For this review, take the finished solid that the model builds, in its own axes (mm). Face numbers are marked on the shaded views. Coordinates: 2 decimals unless noted, no trailing zeros. Loops run counter-clockwise (first coordinate to the right, second up) from the corner with the lowest first, then second, coordinate; pieces in that order, holes last.
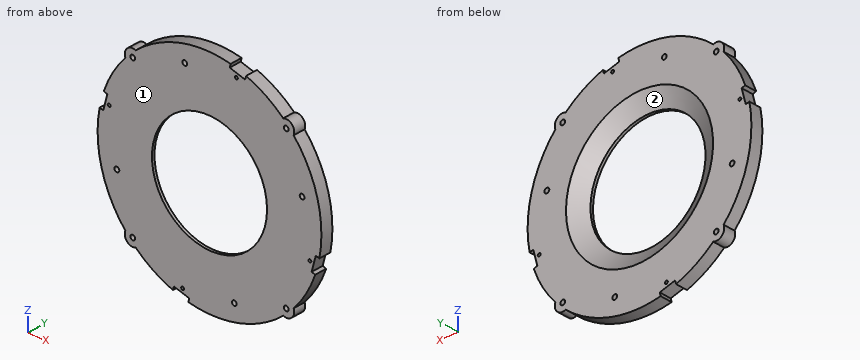
```python
from build123d import *

# Parameters (mm, degrees)
SKETCH1_R           = 1.905
BOSS_EXTRUDE1_DEPTH = 9.525
SKETCH2_R           = 45.72
CUT_EXTRUDE1_DEPTH  = 12.7
SKETCH10_R          = 0.6985
CUT_EXTRUDE5_DEPTH  = 3.175
CIRPATTERN5_COUNT   = 4
CHAMFER1_SIZE       = 12.7
CHAMFER1_SIZE2      = 7.332348419
SKETCH4_R           = 1.905
CUT_EXTRUDE6_DEPTH  = 10.5250001
CIRPATTERN6_COUNT   = 4
SKETCH13_R          = 1.1303
CUT_EXTRUDE7_DEPTH  = 10.5250001
CIRPATTERN7_COUNT   = 4
SKETCH14_W          = 11.95230377
SKETCH14_H          = 12.7
CUT_EXTRUDE8_DEPTH  = 3.175
CIRPATTERN8_COUNT   = 4


with BuildPart() as part:
    # Sketch1 → Boss-Extrude1 (new body)
    with BuildSketch(Plane(origin=(0, 0, 0), x_dir=(1, 0, 0), z_dir=(0, 1, 0))):
        with BuildLine():
            ThreePointArc((-66.860826677, 58.590441679), (-88.9, 0), (-66.860826677, -58.590441679))
            ThreePointArc((-66.860826677, -58.590441679), (-65.466067123, -65.466067123), (-58.590441679, -66.860826677))
            ThreePointArc((-58.590441679, -66.860826677), (0, -88.9), (58.590441679, -66.860826677))
            ThreePointArc((58.590441679, -66.860826677), (65.466067123, -65.466067123), (66.860826677, -58.590441679))
            ThreePointArc((66.860826677, -58.590441679), (88.9, 0), (66.860826677, 58.590441679))
            ThreePointArc((66.860826677, 58.590441679), (65.466067123, 65.466067123), (58.590441679, 66.860826677))
            ThreePointArc((58.590441679, 66.860826677), (0, 88.9), (-58.590441679, 66.860826677))
            ThreePointArc((-58.590441679, 66.860826677), (-65.466067123, 65.466067123), (-66.860826677, 58.590441679))
        make_face()
        with Locations((-60.975939062, 60.975939062)):
            Circle(SKETCH1_R, mode=Mode.SUBTRACT)
        with Locations((60.975939062, 60.975939062)):
            Circle(SKETCH1_R, mode=Mode.SUBTRACT)
        with Locations((60.975939062, -60.975939062)):
            Circle(SKETCH1_R, mode=Mode.SUBTRACT)
        with Locations((-60.975939062, -60.975939062)):
            Circle(SKETCH1_R, mode=Mode.SUBTRACT)
    extrude(amount=BOSS_EXTRUDE1_DEPTH)

    # Sketch2 → Cut-Extrude1 (cut)
    with BuildSketch(Plane(origin=(0, 9.525, 0), x_dir=(1, 0, 0), z_dir=(0, 1, 0))):
        Circle(SKETCH2_R)
    extrude(amount=-CUT_EXTRUDE1_DEPTH, mode=Mode.SUBTRACT)

    # Sketch10 → Cut-Extrude5 (cut)
    with BuildSketch(Plane(origin=(-62.861792847, 0, -62.861792847), x_dir=(0, -1, 0), z_dir=(-0.707106781, 0, -0.707106781))):
        with Locations((-4.826, 0)):
            Circle(SKETCH10_R)
    cut_extrude5 = extrude(amount=-CUT_EXTRUDE5_DEPTH, mode=Mode.SUBTRACT)

    # CirPattern5: Cut-Extrude5 ×4 about axis
    cirpattern5_axis = Axis((0, 0, 0), (0, 1, 0))
    for i in range(1, CIRPATTERN5_COUNT):
        add(cut_extrude5.rotate(cirpattern5_axis, i * 360 / CIRPATTERN5_COUNT), mode=Mode.SUBTRACT)

    # Chamfer1
    chamfer1_edges = [part.edges().sort_by_distance(p)[0] for p in [
        (-45.72, 9.525, 0),
    ]]
    chamfer1_side = [part.faces().sort_by_distance(p)[0] for p in [
        (0, 9.525, -86.385528286),
    ]]
    chamfer(chamfer1_edges, length=CHAMFER1_SIZE, length2=CHAMFER1_SIZE2, reference=chamfer1_side[0])

    # Sketch4 → Cut-Extrude6 (cut, through all)
    with BuildSketch(Plane(origin=(0, 9.525, 0), x_dir=(1, 0, 0), z_dir=(0, 1, 0))):
        with Locations((19.722011237, 73.603547963)):
            Circle(SKETCH4_R)
    cut_extrude6 = extrude(amount=-CUT_EXTRUDE6_DEPTH, mode=Mode.SUBTRACT)

    # CirPattern6: Cut-Extrude6 ×4 about axis
    cirpattern6_axis = Axis((0, 0, 0), (0, 1, 0))
    for i in range(1, CIRPATTERN6_COUNT):
        add(cut_extrude6.rotate(cirpattern6_axis, i * 360 / CIRPATTERN6_COUNT), mode=Mode.SUBTRACT)

    # Sketch13 → Cut-Extrude7 (cut, through all)
    with BuildSketch(Plane(origin=(0, 9.525, 0), x_dir=(1, 0, 0), z_dir=(0, 1, 0))):
        with Locations((-21.365512173, 79.73717696)):
            Circle(SKETCH13_R)
    cut_extrude7 = extrude(amount=-CUT_EXTRUDE7_DEPTH, mode=Mode.SUBTRACT)

    # CirPattern7: Cut-Extrude7 ×4 about axis
    cirpattern7_axis = Axis((0, 0, 0), (0, 1, 0))
    for i in range(1, CIRPATTERN7_COUNT):
        add(cut_extrude7.rotate(cirpattern7_axis, i * 360 / CIRPATTERN7_COUNT), mode=Mode.SUBTRACT)

    # Sketch14 → Cut-Extrude8 (cut)
    with BuildSketch(Plane(origin=(-23.00901311, 0, -85.870805957), x_dir=(0, -1, 0), z_dir=(-0.258819045, 0, -0.965925826))):
        with Locations((-4.621692603, 0)):
            Rectangle(SKETCH14_W, SKETCH14_H)
    cut_extrude8 = extrude(amount=-CUT_EXTRUDE8_DEPTH, mode=Mode.SUBTRACT)

    # CirPattern8: Cut-Extrude8 ×4 about axis
    cirpattern8_axis = Axis((0, 0, 0), (0, 1, 0))
    for i in range(1, CIRPATTERN8_COUNT):
        add(cut_extrude8.rotate(cirpattern8_axis, i * 360 / CIRPATTERN8_COUNT), mode=Mode.SUBTRACT)


solid = part.part
```
Q1. Consider section B-B (z = 0). State the section outline as (x, y) points (3 decimals), then the cut area to 3 significant figures.
Q2. The part is to be moulded in two halves that separate along Z. For the marked faces 1 and 2, say which applies: +Z half, -Z half, draft (parallel to the pull), parting line (faces both ways), or undercut.
Q3. Wall thickness on probe 1 along X at (y, z) = (0.5, 39.5); probe 2 along X at (y, z) = (5, -11); probe 3 along Z at (x, y) = (-33, 8.5): over which ranges is each line inside the solid? List them lowest first.
Q4. Consider section A-A (x = 0). State the section outline as (y, z) points (3 decimals), then the cut area to 3 significant figures.
Q5. For pin 1 Ø1 at (x, y) = (-60.5, 1) entering from -Z; pin 2 Ø1.5 at (x, y) = (-18, 3.5) entering from +Z; pin 3 Ø4 at (y, z) = (6, -8) entering from +X, all flat-tipped, find the tip position at first contact; note any pin that passes through.
Model answer:
1. outline: (-88.9, 0) - (-45.72, 0) - (-45.72, 2.193) - (-58.42, 9.525) - (-88.9, 9.525) - close; (45.72, 0) - (88.9, 0) - (88.9, 9.525) - (58.42, 9.525) - (45.72, 2.193) - close
1. area: 729 mm2
2. face 1: draft
2. face 2: undercut
3. probe 1: x = -79.64 to -23.02, 23.02 to 79.64
3. probe 2: x = -88.22 to -49.37, 49.37 to 88.22
3. probe 3: z = -82.55 to -46.04, 46.04 to 82.55
4. outline: (0, -88.9) - (9.525, -88.9) - (9.525, -58.42) - (2.193, -45.72) - (0, -45.72) - close; (0, 45.72) - (2.193, 45.72) - (9.525, 58.42) - (9.525, 88.9) - (0, 88.9) - close
4. area: 729 mm2
5. pin 1: stops at z = -67.33
5. pin 2: stops at z = 87.21
5. pin 3: stops at x = 88.7
